The model under review builds one solid part; all positions refer to its coordinate system, in mm. A direction names the side the tool comes from. Give positions to 0.01 mm unless a question says otherwise; leave off trailing zeros. Write each loop counter-clockwise with the first axis right and the second up, starting at its lowest first coordinate (ties: lowest second). Pieces come first, ordered by that corner, then holes.
from build123d import *
from build123d.topology import SkipClean

# Parameters (mm, degrees)
SKETCH1_R               = 34.1
BOSS_EXTRUDE1_DEPTH     = 1.75
SKETCH4_R               = 28.5
BOSS_EXTRUDE2_DEPTH     = 2
SKETCH5_R               = 34.1
SKETCH5_R_2             = 16.25
BOSS_EXTRUDE3_DEPTH     = 5
CUT_EXTRUDE2_DEPTH      = 49.968050809
CUT_EXTRUDE2_DEPTH_BACK = 49.968050809
SKETCH3_R               = 2.25
CUT_EXTRUDE1_DEPTH      = 49.968050809
CUT_EXTRUDE1_DEPTH_BACK = 49.968050809
SKETCH2_R               = 7.25
SKETCH6_R               = 2.25
CUT_EXTRUDE3_DEPTH      = 50.354533733
CIRPATTERN1_COUNT       = 8
SKETCH7_R               = 20.5
SKETCH7_R_2             = 2.25
SKETCH7_R_3             = 7.25
BOSS_EXTRUDE4_DEPTH     = 5
BOSS_EXTRUDE5_START     = 2
SKETCH8_R               = 34.1
SKETCH8_R_2             = 28.5
BOSS_EXTRUDE5_DEPTH     = 2
SKETCH10_R              = 34.1
SKETCH10_R_2            = 20.5
CUT_EXTRUDE4_DEPTH      = 2
CUT_EXTRUDE5_DEPTH      = 4
SKETCH12_R              = 4.6
CUT_EXTRUDE6_DEPTH      = 3
FILLET2_R               = 1
FILLET3_R               = 1


with BuildPart() as part:
    # Sketch1 → Boss-Extrude1 (new, symmetric)
    with BuildSketch(Plane.XY):
        Circle(SKETCH1_R)
    extrude(amount=BOSS_EXTRUDE1_DEPTH, both=True)

    # Sketch4 → Boss-Extrude2 (add)
    with BuildSketch(Plane.XY.offset(1.75)):
        Circle(SKETCH4_R)
    extrude(amount=BOSS_EXTRUDE2_DEPTH)

    # Sketch5 → Boss-Extrude3 (add)
    with BuildSketch(Plane(origin=(0, 0, -1.75), x_dir=(-1, 0, 0), z_dir=(0, 0, -1))):
        Circle(SKETCH5_R)
        Circle(SKETCH5_R_2, mode=Mode.SUBTRACT)
    extrude(amount=BOSS_EXTRUDE3_DEPTH)

    # Sketch3 → Cut-Extrude2 (cut, two sides: drawn at the far end of the back side and taken through both)
    with BuildSketch(Plane.XY.offset(1.75).offset(-CUT_EXTRUDE2_DEPTH_BACK)):
        with Locations((0, 11.3137085)):
            Circle(SKETCH3_R)
        with Locations((11.3137085, 0)):
            Circle(SKETCH3_R)
        with Locations((0, -11.3137085)):
            Circle(SKETCH3_R)
        with Locations((-11.3137085, 0)):
            Circle(SKETCH3_R)
    extrude(amount=CUT_EXTRUDE2_DEPTH + CUT_EXTRUDE2_DEPTH_BACK, mode=Mode.SUBTRACT)

    # Sketch2 → Cut-Extrude1 (cut, two sides: drawn at the far end of the back side and taken through both)
    with BuildSketch(Plane.XY.offset(1.75).offset(-CUT_EXTRUDE1_DEPTH_BACK)):
        Circle(SKETCH2_R)
    extrude(amount=CUT_EXTRUDE1_DEPTH + CUT_EXTRUDE1_DEPTH_BACK, mode=Mode.SUBTRACT)

    # Sketch6 → Cut-Extrude3 (cut, symmetric)
    with BuildSketch(Plane.XY.offset(3.75)):
        with Locations((0, 24.75)):
            Circle(SKETCH6_R)
    cut_extrude3 = extrude(amount=CUT_EXTRUDE3_DEPTH, both=True, mode=Mode.SUBTRACT)

    # CirPattern1: Cut-Extrude3 ×8 about axis
    cirpattern1_axis = Axis((0, 0, 0), (0, 0, 1))
    for i in range(1, CIRPATTERN1_COUNT):
        add(cut_extrude3.rotate(cirpattern1_axis, i * 360 / CIRPATTERN1_COUNT), mode=Mode.SUBTRACT)

    # Sketch7 → Boss-Extrude4 (add)
    with BuildSketch(Plane.XY.offset(3.75)):
        Circle(SKETCH7_R)
        with Locations((0, -11.3137085)):
            Circle(SKETCH7_R_2, mode=Mode.SUBTRACT)
        with Locations((11.3137085, 0)):
            Circle(SKETCH7_R_2, mode=Mode.SUBTRACT)
        with Locations((0, 11.3137085)):
            Circle(SKETCH7_R_2, mode=Mode.SUBTRACT)
        with Locations((-11.3137085, 0)):
            Circle(SKETCH7_R_2, mode=Mode.SUBTRACT)
        Circle(SKETCH7_R_3, mode=Mode.SUBTRACT)
    extrude(amount=BOSS_EXTRUDE4_DEPTH)

    # Sketch8 → Boss-Extrude5 (add)
    with SkipClean():  # the faces are left unmerged after this step: merging them gives an invalid solid
        with BuildSketch(Plane.XY.offset(1.75).offset(BOSS_EXTRUDE5_START)):
            with Locations(Location((0, 0, 0), (0, 0, 180))):
                Circle(SKETCH8_R)
            Circle(SKETCH8_R_2, mode=Mode.SUBTRACT)
        extrude(amount=-BOSS_EXTRUDE5_DEPTH)

    # Sketch10 → Cut-Extrude4 (cut)
    with BuildSketch(Plane.XY.offset(3.75)):
        with Locations(Location((0, 0, 0), (0, 0, 180))):
            Circle(SKETCH10_R)
        Circle(SKETCH10_R_2, mode=Mode.SUBTRACT)
    extrude(amount=-CUT_EXTRUDE4_DEPTH, mode=Mode.SUBTRACT)

    # Sketch11 → Cut-Extrude5 (cut)
    with BuildSketch(Plane.XY.offset(8.75)):
        with BuildLine():
            Line((-11.3137085, 3.6), (-8.248636251, 3.6))
            ThreePointArc((-8.248636251, 3.6), (-6.363961031, 6.363961031), (-3.6, 8.248636251))
            Line((-3.6, 8.248636251), (-3.6, 11.3137085))
            ThreePointArc((-3.6, 11.3137085), (0, 14.9137085), (3.6, 11.3137085))
            Line((3.6, 11.3137085), (3.6, 8.248636251))
            ThreePointArc((3.6, 8.248636251), (6.363961031, 6.363961031), (8.248636251, 3.6))
            Line((8.248636251, 3.6), (11.3137085, 3.6))
            ThreePointArc((11.3137085, 3.6), (14.9137085, 0), (11.3137085, -3.6))
            Line((11.3137085, -3.6), (8.248636251, -3.6))
            ThreePointArc((8.248636251, -3.6), (6.363961031, -6.363961031), (3.6, -8.248636251))
            Line((3.6, -8.248636251), (3.6, -11.3137085))
            ThreePointArc((3.6, -11.3137085), (0, -14.9137085), (-3.6, -11.3137085))
            Line((-3.6, -11.3137085), (-3.6, -8.248636251))
            ThreePointArc((-3.6, -8.248636251), (-6.363961031, -6.363961031), (-8.248636251, -3.6))
            Line((-8.248636251, -3.6), (-11.3137085, -3.6))
            ThreePointArc((-11.3137085, -3.6), (-14.9137085, 0), (-11.3137085, 3.6))
        make_face()
    extrude(amount=-CUT_EXTRUDE5_DEPTH, mode=Mode.SUBTRACT)

    # Sketch12 → Cut-Extrude6 (cut)
    with BuildSketch(Plane(origin=(0, 0, -6.75), x_dir=(-1, 0, 0), z_dir=(0, 0, -1))):
        with Locations((0, 24.75)):
            Circle(SKETCH12_R)
        with Locations((17.500892834, 17.500892834)):
            Circle(SKETCH12_R)
        with Locations((24.75, 0)):
            Circle(SKETCH12_R)
        with Locations((17.500892834, -17.500892834)):
            Circle(SKETCH12_R)
        with Locations((0, -24.75)):
            Circle(SKETCH12_R)
        with Locations((-17.500892834, -17.500892834)):
            Circle(SKETCH12_R)
        with Locations((-24.75, 0)):
            Circle(SKETCH12_R)
        with Locations((-17.500892834, 17.500892834)):
            Circle(SKETCH12_R)
    extrude(amount=-CUT_EXTRUDE6_DEPTH, mode=Mode.SUBTRACT)

    # Fillet2
    fillet2_edges = [part.edges().sort_by_distance(p)[0] for p in [
        (-20.5, 0, 8.75),
    ]]
    fillet(fillet2_edges, radius=FILLET2_R)

    # Fillet3
    fillet3_edges = [part.edges().sort_by_distance(p)[0] for p in [
        (16.25, 0, -1.75),
    ]]
    fillet(fillet3_edges, radius=FILLET3_R)


solid = part.part
1) Consider section B-B, the plane x = -24.75. Give the boundary of the cut face in (y, z).
2) Insertion check: pin 1 (6 mm diameter, centred on x = -17.5, y = -17.5, fed in from -Z); pin 2 (5.5 mm diameter, centred on x = -17.5, y = 17.5, fed in from +Z); pin 3 (2.5 mm diameter, centred on x = -10, z = 6, fed in from +Y). Each pin has a flat end and moves straight along its axis. Give the tip position at first contact, or say it passes through.
3) To check wall thickness, follow probe 1 along Y at (x, z) = (0, -6); probe 2 along Y at (x, z) = (0, 1.25); probe 3 along X at (y, z) = (1.5, -5.5). State the ranges of each line that lie inside material, in increasing order.
4) Consider section A-A, the plane y = 0. State how many separate pieces and enclosed holes the cut face has, then the cut area to 3 significant figures.
5) The part is to be moulded in two halves that separate along Y. For faces 4 (the flat face through (20, 17, -3.75)), 5 (the flat face through (8.4, -4.1, 8.75)), say which applies: +Y half, -Y half, draft (parallel to the pull), parting line (faces both ways), or undercut.
6) Tool access review of faces 1 (the cylindrical face through (22.554, 0.488, -0.962)), 2 (the cylindrical face through (-15.5, 4.88, -4.72)), 3 (the cylindrical face through (0.079, -14.913, 6.778)): name each direction out of +Z, -Z, +X, -X, +Y, -Y from which nothing blocks a thin tool from reaching the whole face with its end or side.
Answer block:
1. outline: (-23.46, -6.75) - (-4.6, -6.75) - (-4.6, -3.75) - (-2.25, -3.75) - (-2.25, 1.75) - (-23.46, 1.75) - close; (2.25, -3.75) - (4.6, -3.75) - (4.6, -6.75) - (23.46, -6.75) - (23.46, 1.75) - (2.25, 1.75) - close
2. pin 1: stops at z = -3.75
2. pin 2: stops at z = 1.75
2. pin 3: stops at y = 18.54
3. probe 1: y = -34.1 to -29.35, -20.15 to -16.25, 16.25 to 20.15, 29.35 to 34.1
3. probe 2: y = -34.1 to -27, -22.5 to -13.56, -9.06 to -7.25, 7.25 to 9.06, 13.56 to 22.5, 27 to 34.1
3. probe 3: x = -34.07 to -29.1, -20.4 to -16.18, 16.18 to 20.4, 29.1 to 34.07
4. separate pieces: 6
4. enclosed holes: 0
4. area: 327 mm2
5. face 4: undercut
5. face 5: draft
6. face 1: +Z, -Z
6. face 2: -Z
6. face 3: +Z
